from build123d import *

# Parameters (mm, degrees)
RESSALTO_EXTRUS_O2_DEPTH = 9
CASCA1_T                 = -3
CHANFRO1_SIZE            = 3


with BuildPart() as part:
    # Esboço1 → Ressalto-extrusão2 (new body)
    with BuildSketch(Plane(origin=(0, 0, 0), x_dir=(1, 0, 0), z_dir=(0, 1, 0))):
        Polygon((30.237590053, -73), (73, -30.237590053), (73, 30.237590053), (30.237590053, 73), (-30.237590053, 73), (-73, 30.237590053), (-73, -30.237590053), (-30.237590053, -73), align=None)
    extrude(amount=RESSALTO_EXTRUS_O2_DEPTH)

    # Casca1
    casca1_openings = [part.faces().sort_by_distance(p)[0] for p in [
        (0, 0, 0),
    ]]
    offset(amount=CASCA1_T, openings=casca1_openings, kind=Kind.INTERSECTION)

    # Chanfro1
    chanfro1_edges = [part.edges().sort_by_distance(p)[0] for p in [
        (73, 9, 0),
        (51.618795027, 9, -51.618795027),
        (0, 9, -73),
        (-51.618795027, 9, -51.618795027),
        (-73, 9, 0),
        (-51.618795027, 9, 51.618795027),
        (0, 9, 73),
        (51.618795027, 9, 51.618795027),
    ]]
    chamfer(chanfro1_edges, length=CHANFRO1_SIZE)


solid = part.part
Read the model definition and answer for the solid it produces. Units are mm, in the model's axes. A direction names the side the tool comes from. Coordinates: 2 decimals unless noted, no trailing zeros. Order: outer loops, then holes, each group sorted by start corner. A loop starts at its lowest first (then second) coordinate and runs counter-clockwise, first axis right, second up. Notation, with made-up numbers: (80.25, 71.5) -> (128.25, 71.5) arc R27 cw to (128.25, 102.5) -> close; hole circle Ø11 at (-8.5, -2.75). An arc over 180 degrees is marked (long way). Answer as a JSON object with one key per item and string values.
1) A tool of negligible diameter and unlimited length cuts with its end or side. For faces 1 (the face through (0, 3, -70)), 2 (the face through (73, 3, 0)), from which of +Z, -Z, +X, -X, +Y, -Y can it reach the whole face along a straight path? Write none if from no direction.
Model answer:
{"face 1": "-Y", "face 2": "+Z, -Z, +X, +Y, -Y"}
2) Each of these flat-tipped pins is pushed along its axis until it touches: pin 1 (2 mm diameter, centred on x = 42.5, y = 2, fed in from +Z); pin 2 (5 mm diameter, centred on x = 9, z = -13, fed in from -Y); pin 3 (3 mm diameter, centred on y = 5, z = -38.5, fed in from -X). Where does it stop, or does it pass through?
Model answer:
{"pin 1": "stops at z = 61.74", "pin 2": "stops at y = 6", "pin 3": "stops at x = -66.24"}
3) A cutting plane is placed at C-C, the plane x = -16.5. Determine the outline of the cut face in (y, z), plus the area to 3 significant figures.
Model answer:
{"outline": "(0, -73) -> (6, -73) -> (9, -70) -> (9, 70) -> (6, 73) -> (0, 73) -> (0, 70) -> (6, 70) -> (6, -70) -> (0, -70) -> close", "area": "465 mm²"}
4) A cutting plane is placed at B-B, the plane y = 2.5. Determine the outline of the cut face in (x, z), plus the area to 3 significant figures.
Model answer:
{"outline": "(-73, -30.24) -> (-30.24, -73) -> (30.24, -73) -> (73, -30.24) -> (73, 30.24) -> (30.24, 73) -> (-30.24, 73) -> (-73, 30.24) -> close; hole (-70, -28.99) -> (-28.99, -70) -> (28.99, -70) -> (70, -28.99) -> (70, 28.99) -> (28.99, 70) -> (-28.99, 70) -> (-70, 28.99) -> close", "area": "1,420 mm²"}
5) Consider line 1 along X through (y, z) = (1, -4.5); line 2 along Y through (x, z) = (-40.5, 14). Determine where each line is inside the solid, lowest interval first. Write a range as from..to.
Model answer:
{"line 1": "x = -73..-70, 70..73", "line 2": "y = 6..9"}
6) The mould has two halves that part along X. Classify faces 3 (the face through (0, 3, -73)), 4 (the face through (49.21, 2.958, 49.785)), 5 (the face through (51.32, 2.96, 51.92)): released by +X, released by -X, zero draft, split by the parting line, or undercut.
Model answer:
{"face 3": "zero draft", "face 4": "undercut", "face 5": "released by +X"}
7) A cutting plane is placed at A-A, the plane z = -7.5. Determine the outline of the cut face in (x, y).
Model answer:
{"outline": "(-73, 0) -> (-70, 0) -> (-70, 6) -> (70, 6) -> (70, 0) -> (73, 0) -> (73, 6) -> (70, 9) -> (-70, 9) -> (-73, 6) -> close"}
